Build history of the part. All positions in model axes, mm. A direction names the side the tool comes from. Give positions to 0.01 mm unless a question says otherwise; leave off trailing zeros. Order: outer loops, then holes, each group sorted by start corner. A loop starts at its lowest first (then second) coordinate and runs counter-clockwise, first axis right, second up. Notation, with made-up numbers: (-12, 32) -> (14, 32) arc R15 cw to (14, 57) -> close; hole circle Ø2 at (-38.5, 36). An arc over 180 degrees is marked (long way). One line per item, written item: value. Start each with the question number.
(1) Probe line 1 (Z direction, x = -7.25, y = 9.5); line 2 (Y direction, x = -11.75, z = -91); line 3 (Y direction, x = -8.5, z = -100). List the from-to ranges inside material, lowest first.
(2) Saw through at B-B on x = -8.25. Give the cut face in (y, z), plus the area to 3 significant figures.
(3) Which spindle directions (+Z, -Z, +X, -X, +Y, -Y) get a long thin tool onto all of the face, cutting with end or side? Do faces 1 (the flat face through (-8, 61, -12)), 2 (the cylindrical face through (-7.281, 57.594, -5.916)), 3 (the flat face through (-3, 36, -17)), 4 (the cylindrical face through (-7.406, 4.056, -19.281)). Say none if no direction does.
(4) Two-plate mould, pull along Z, no slides. Class faces 5 (the flat face through (-3, 36, -87)), 6 (the flat face through (-4, 35, -104)), 7 (the flat face through (0, 11, -51)): +Z half, -Z half, draft (parallel to the pull), parting line (faces both ways), or undercut.
(5) Pin check, flat tips, straight feed: pin 1 (4 mm diameter, centred on y = 66, z = -98, fed in from -X); pin 2 (5 mm diameter, centred on x = -6.5, y = 39.5, fed in from +Z); pin 3 (8 mm diameter, centred on y = 43, z = -19.5, fed in from -X). Stop position of each tip, or through.
(6) Saw through at A-A on z = -98. Count the separate pieces of the cut face and the enclosed holes in it, plus the area to 3 significant figures.
(7) Saw through at C-C on z = -35. Give the cut face in (x, y), plus the area to 3 significant figures.
(8) Saw through at D-D on y = 49. Give the cut face in (x, z).
Autodesk Inventor part; units mm, degrees
ref_plane "YZ Plane" through (0, 0, 0) normal (1, 0, 0) x (0, 1, 0)
ref_plane "XZ Plane" through (0, 0, 0) normal (0, 1, 0) x (-1, 0, 0)
ref_plane "XY Plane" through (0, 0, 0) normal (0, 0, 1) x (1, 0, 0)
sketch "Sketch1" plane through (0, 0, 0) normal (0, 1, 0) x (-1, 0, 0)
  line L0 (0, 0) -> (0, -104)
  line L1 (0, 0) -> (13, 0)
  line L2 (13, 0) -> (13, -12)
  line L3 (13, -12) -> (5, -12)
  line L4 (5, -12) -> (5, -92)
  line L5 (5, -92) -> (13, -92)
  line L6 (13, -92) -> (13, -104)
  line L7 (13, -104) -> (0, -104)
  dimension "d0" = 104
  dimension "d1" = 13
  dimension "d2" = 12
  dimension "d3" = 8
  dimension "d4" = 80
  dimension "d5" = 8
extrude "Extrusion1" add sketch "Sketch1" along normal blind 72
sketch "Sketch3" plane through (-5, 0, -92) normal (-1, 0, 0) x (0, 0, 1)
  line L0 (0, 0) -> (80, 0)
  line L1 (0, 0) -> (80, 0)
  line L2 (80, 0) -> (80, 72)
  line L3 (0, 72) -> (80, 72)
  line L4 (0, 0) -> (0, 72)
  line L5 (0, 0) -> (0, 72)
  line L6 (80, 0) -> (0, 0)
  line L7 (0, 0) -> (0, 8)
  line L8 (0, 8) -> (80, 8)
  line L9 (80, 8) -> (80, 0)
  line L10 (80, 0) -> (80, 72)
  line L11 (80, 72) -> (0, 72)
  line L12 (0, 72) -> (0, 64)
  line L13 (0, 64) -> (80, 64)
  line L14 (80, 64) -> (80, 72)
  point P0 (92, 0)
  dimension "d14" = 8
  dimension "d15" = 8
extrude "Extrusion3" add sketch "Sketch3" along normal blind 8 contours L4 L8 L2 L0 | L4 L3 L2 L13
sketch "Sketch4" plane through (-13, 0, -104) normal (-1, 0, 0) x (0, 0, 1)
  circle A0 centre (98, 66) radius 2.5
  line L0 (0, 72) -> (104, 72)
  line L1 (0, 0) -> (0, 72)
  line L2 (0, 0) -> (104, 0)
  line L3 (104, 0) -> (104, 72)
  line L4 (12, 64) -> (92, 64)
  line L5 (92, 8) -> (92, 64)
  line L6 (92, 8) -> (12, 8)
  line L7 (12, 8) -> (12, 64)
  circle A1 centre (6, 6) radius 2.5
  circle A2 centre (98, 6) radius 2.5
  circle A3 centre (6, 66) radius 2.5
  line L8 (0, 0) -> (0, 72)
  line L9 (104, 0) -> (104, 72)
  dimension "d18" = 5
  dimension "d19" = 6
  dimension "d20" = 6
  dimension "d25" = 5
  dimension "d31" = 5
  dimension "d32" = 5
  dimension "d37" = 6
  dimension "d38" = 6
  dimension "d46" = 6
  dimension "d47" = 6
extrude "Extrusion5" cut sketch "Sketch4" against normal through all contours A0 | A1 | A2 | A3
sketch "Sketch5" plane through (-5, 8, -92) normal (-1, 0, 0) x (0, 0, 1)
  line L0 (80, 0) -> (0, 0)
  line L1 (5, 5) -> (75, 5)
  line L2 (75, 5) -> (75, 51)
  line L3 (75, 51) -> (5, 51)
  line L4 (5, 51) -> (5, 5)
  line L5 (0, 0) -> (0, 56)
  line L6 (80, 56) -> (0, 56)
  line L7 (0, 0) -> (0, 56)
  line L8 (0, 0) -> (80, 0)
  line L9 (80, 0) -> (80, 56)
  line L10 (0, 56) -> (80, 56)
  line L11 (80, 0) -> (80, 56)
  point P0 (92, -8)
  dimension "d50" = 5
  dimension "d51" = 5
  dimension "d52" = 5
  dimension "d53" = 5
extrude "Extrusion6" cut sketch "Sketch5" against normal through all contours L4 L3 L2 L1
sketch "Sketch6" plane through (-13, 0, -104) normal (-1, 0, 0) x (0, 0, 1)
  line L0 (92, 8) -> (92, 64)
  line L1 (92, 12) -> (104, 12)
  line L2 (104, 0) -> (104, 72)
  line L3 (92, 60) -> (104, 60)
  line L4 (12, 8) -> (12, 64)
  line L5 (12, 12) -> (0, 12)
  line L6 (0, 0) -> (0, 72)
  line L7 (12, 60) -> (0, 60)
  line L8 (0, 72) -> (104, 72)
  line L9 (0, 0) -> (104, 0)
  line L10 (0, 12) -> (0, 60)
  line L11 (12, 12) -> (12, 60)
  line L12 (92, 12) -> (92, 60)
  line L13 (104, 12) -> (104, 60)
  dimension "d56" = 12
  dimension "d57" = 12
extrude "Extrusion7" cut sketch "Sketch6" against normal blind 8 contours L0 L3 L2 L1 | L6 L7 L4 L5
fillet "Fillet1" radius 8 1 edges at (-5, 12, -98)
fillet "Fillet2" radius 8 1 edges at (-5, 60, -98)
fillet "Fillet3" radius 8 2 edges at (-5, 12, -6) (-5, 60, -6)
sketch "Sketch7" plane through (-13, 72, -104) normal (-1, 0, 0) x (0, 0, 1)
  line L0 (104, 0) -> (0, 0)
  line L1 (17, -72) -> (87, -72)
  line L2 (87, -72) -> (87, 0)
  line L3 (87, 0) -> (17, 0)
  line L4 (17, 0) -> (17, -72)
  line L5 (0, -72) -> (0, -60)
  point P0 (104, -72)
  dimension "d63" = 17
  dimension "d64" = 17
  dimension "d65" = 72
extrude "Extrusion8" cut sketch "Sketch7" against normal blind 8
fillet "Fillet4" radius 8 4 edges at (-5, 4, -87) (-5, 68, -87) (-5, 4, -17) (-5, 68, -17)
properties part number "batteryholder"
Results below:
1. line 1: z = -104 to -92, -12 to 0
1. line 2: y = 0 to 8, 64 to 72
1. line 3: y = 0 to 4.5, 7.5 to 13.39, 58.61 to 64.5, 67.5 to 72
2. outline: (0, -104) -> (13.56, -104) -> (13.56, -92) -> (8, -92) -> (8, -85.44) -> (0, -85.44) -> close; (0, -18.56) -> (8, -18.56) -> (8, -12) -> (13.56, -12) -> (13.56, 0) -> (0, 0) -> close; (58.44, -104) -> (72, -104) -> (72, -85.44) -> (64, -85.44) -> (64, -92) -> (58.44, -92) -> close; (58.44, -12) -> (64, -12) -> (64, -18.56) -> (72, -18.56) -> (72, 0) -> (58.44, 0) -> close; hole circle Ø5 at (6, -98); hole circle Ø5 at (6, -6); hole circle Ø5 at (66, -98); hole circle Ø5 at (66, -6)
2. area: 782 mm²
3. face 1: -X
3. face 2: +Z, -Z, -X
3. face 3: +X, -X
3. face 4: -X, +Y, -Y
4. face 5: undercut
4. face 6: -Z half
4. face 7: draft
5. pin 1: passes through
5. pin 2: stops at z = 0
5. pin 3: stops at x = -5
6. separate pieces: 3
6. enclosed holes: 0
6. area: 449 mm²
7. outline: (-5, 0) -> (0, 0) -> (0, 13) -> (-5, 13) -> close; (-5, 59) -> (0, 59) -> (0, 72) -> (-5, 72) -> close
7. area: 130 mm²
8. outline: (-5, -104) -> (0, -104) -> (0, -87) -> (-5, -87) -> close; (-5, -17) -> (0, -17) -> (0, 0) -> (-5, 0) -> close
